```python
from build123d import *

# Parameters (mm, degrees)
SKETCH_1_W             = 94
SKETCH_1_H             = 94
EXTRUDE_1_DEPTH        = 30
FILLET_1_R             = 10
SHELL_1_T              = -2
SKETCH_2_W             = 24.1
SKETCH_2_H             = 30
EXTRUDE_3392_DEPTH     = 11
CUT_EXTRUDE_3513_REACH = 111.293
SKETCH_3_W             = 18.42
SKETCH_3_H             = 11.6
SKETCH_4_W             = 24.1
SKETCH_4_H             = 24.1
CUT_EXTRUDE_3826_DEPTH = 1.4
EXTRUDE_4548_DEPTH     = 14.2
SKETCH_9_W             = 69.4
SKETCH_9_H             = 9.2
SKETCH_10_W            = 5
SKETCH_10_H            = 5
EXTRUDE_5202_DEPTH     = 24.19
CUT_EXTRUDE_5310_DEPTH = 4
USBC_REACH             = 111.293
USBC_2_DEPTH           = 26
SKETCH_22_W            = 24.1
SKETCH_22_H            = 10.2
EXTRUDE_7617_DEPTH     = 24.95
CUT_EXTRUDE_6_REACH    = 70.81
SKETCH_23_R            = 2.2
SKETCH_23_R_2          = 3.7
SKETCH_13_W            = 10.3
SKETCH_13_H            = 10.3
EXTRUDE_4_DEPTH        = 28
CUT_EXTRUDE_7_DEPTH    = 4


with BuildPart() as part:
    # 草图1 → 凸台-拉伸1 (new body)
    with BuildSketch(Plane(origin=(0, 0, 0), x_dir=(1, 0, 0), z_dir=(0, 1, 0))):
        Rectangle(SKETCH_1_W, SKETCH_1_H)
    extrude(amount=EXTRUDE_1_DEPTH)

    # 圆角1
    fillet_1_edges = [part.edges().sort_by_distance(p)[0] for p in [
        (-47, 15, -47),
        (47, 15, -47),
        (47, 15, 47),
        (-47, 15, 47),
    ]]
    fillet(fillet_1_edges, radius=FILLET_1_R)

    # 抽壳1
    shell_1_openings = [part.faces().sort_by_distance(p)[0] for p in [
        (0, 0, 0),
    ]]
    offset(amount=SHELL_1_T, openings=shell_1_openings, kind=Kind.INTERSECTION)

    # 草图2 → Extrude 3392 (add)
    with BuildSketch(Plane.XY.offset(47)):
        with Locations((0, 15)):
            Rectangle(SKETCH_2_W, SKETCH_2_H)
    extrude(amount=-EXTRUDE_3392_DEPTH)

    # 草图3 → Cut-Extrude 3513 (cut, up to next)
    with BuildSketch(Plane.XY.offset(47), mode=Mode.PRIVATE) as cut_extrude_3513_sk1:
        with Locations((0, 12)):
            Rectangle(SKETCH_3_W, SKETCH_3_H)
    cut_extrude_3513_tool1 = extrude(cut_extrude_3513_sk1.sketch, amount=-CUT_EXTRUDE_3513_REACH, mode=Mode.PRIVATE) & part.part
    add(cut_extrude_3513_tool1.solids().sort_by_distance((0, 12, 47))[0], mode=Mode.SUBTRACT)

    # 草图4 → Cut-Extrude 3826 (cut)
    with BuildSketch(Plane.XZ.offset(-28)):
        with Locations((0, -1)):
            Rectangle(SKETCH_4_W, SKETCH_4_H)
    extrude(amount=-CUT_EXTRUDE_3826_DEPTH, mode=Mode.SUBTRACT)

    # 草图6 → Extrude 4548 (add)
    with BuildSketch(Plane.XZ.offset(-28)):
        with BuildLine():
            Line((-45, -37), (-45, -21.630094022))
            Line((-45, -21.630094022), (45, -21.630094022))
            Line((45, -21.630094022), (45, -37))
            ThreePointArc((45, -37), (42.656854249, -42.656854249), (37, -45))
            Line((37, -45), (-37, -45))
            ThreePointArc((-37, -45), (-42.656854249, -42.656854249), (-45, -37))
        make_face()
    extrude(amount=EXTRUDE_4548_DEPTH)

    # 草图9 → Cut-Revolve 4776 (revolve, cut)
    with BuildSketch(Plane.XZ.offset(-13.8)):
        with Locations((0, -31.2)):
            Rectangle(SKETCH_9_W, SKETCH_9_H)
    revolve(axis=Axis((-34.7, 13.8, -35.8), (1, 0, 0)), mode=Mode.SUBTRACT)

    # 草图10 → Extrude 5202 (add)
    with BuildSketch(Plane.XZ.offset(-28)):
        with Locations((-24, 23)):
            Rectangle(SKETCH_10_W, SKETCH_10_H)
        with Locations((24, -9)):
            Rectangle(SKETCH_10_W, SKETCH_10_H)
    extrude(amount=EXTRUDE_5202_DEPTH)

    # 草图11 → Cut-Extrude 5310 (cut)
    with BuildSketch(Plane.XZ.offset(-3.81)):
        Polygon((-23.076239569, 21.4), (-22.152479139, 23), (-23.076239569, 24.6), (-24.923760431, 24.6), (-25.847520861, 23), (-24.923760431, 21.4), align=None)
        Polygon((24.923760431, -10.6), (25.847520861, -9), (24.923760431, -7.4), (23.076239569, -7.4), (22.152479139, -9), (23.076239569, -10.6), align=None)
    extrude(amount=-CUT_EXTRUDE_5310_DEPTH, mode=Mode.SUBTRACT)

    # 草图15 → USBC (cut, up to next)
    with BuildSketch(Plane.XY.offset(47), mode=Mode.PRIVATE) as usbc_sk1:
        with BuildLine():
            Line((21.125, 13.6), (27.925, 13.6))
            ThreePointArc((27.925, 13.6), (29.525, 12), (27.925, 10.4))
            Line((27.925, 10.4), (21.125, 10.4))
            ThreePointArc((21.125, 10.4), (19.525, 12), (21.125, 13.6))
        make_face()
    usbc_tool1 = extrude(usbc_sk1.sketch, amount=-USBC_REACH, mode=Mode.PRIVATE) & part.part
    add(usbc_tool1.solids().sort_by_distance((24.525, 12, 47))[0], mode=Mode.SUBTRACT)

    # 草图16 → USBC 2 (add)
    with BuildSketch(Plane(origin=(0, 0, 45), x_dir=(-1, 0, 0), z_dir=(0, 0, -1))):
        Polygon((-15.225, 13), (-16.025, 13), (-16.025, 14.6), (-18.858333333, 14.6), (-18.858333333, 28), (-15.225, 28), align=None)
        Polygon((-30.191666667, 28), (-33.825, 28), (-33.825, 13), (-33.025, 13), (-33.025, 14.6), (-30.191666667, 14.6), align=None)
    extrude(amount=USBC_2_DEPTH)

    # 草图22 → Extrude 7617 (add)
    with BuildSketch(Plane(origin=(0, 0, 36), x_dir=(-1, 0, 0), z_dir=(0, 0, -1))):
        with Locations((0, 22.9)):
            Rectangle(SKETCH_22_W, SKETCH_22_H)
    extrude(amount=EXTRUDE_7617_DEPTH)

    # 草图23 → 切除-拉伸6 (cut, up to next)
    with BuildSketch(Plane(origin=(0, 17.8, 0), x_dir=(-1, 0, 0), z_dir=(0, -1, 0)), mode=Mode.PRIVATE) as cut_extrude_6_sk1:
        with Locations(Location((0, -32, 0), (0, 0, 180))):
            Circle(SKETCH_23_R)
    cut_extrude_6_tool1 = extrude(cut_extrude_6_sk1.sketch, amount=-CUT_EXTRUDE_6_REACH, mode=Mode.PRIVATE) & part.part
    # 草图23 → 切除-拉伸6 (cut, up to next)
    with BuildSketch(Plane(origin=(0, 17.8, 0), x_dir=(-1, 0, 0), z_dir=(0, -1, 0)), mode=Mode.PRIVATE) as cut_extrude_6_sk2:
        with Locations(Location((0, -22, 0), (0, 0, 180))):
            Circle(SKETCH_23_R_2)
    cut_extrude_6_tool2 = extrude(cut_extrude_6_sk2.sketch, amount=-CUT_EXTRUDE_6_REACH, mode=Mode.PRIVATE) & part.part
    add(cut_extrude_6_tool1.solids().sort_by_distance((0, 17.8, 32))[0], mode=Mode.SUBTRACT)
    add(cut_extrude_6_tool2.solids().sort_by_distance((0, 17.8, 22))[0], mode=Mode.SUBTRACT)

    # 草图13 → 凸台-拉伸4 (add)
    with BuildSketch(Plane.XZ.offset(-28)):
        with BuildLine():
            Line((-45, -37), (-45, -16.768109074))
            Line((-45, -16.768109074), (-34.7, -16.768109074))
            Line((-34.7, -16.768109074), (-34.7, -45))
            Line((-34.7, -45), (-37, -45))
            ThreePointArc((-37, -45), (-42.656854249, -42.656854249), (-45, -37))
        make_face()
        with BuildLine():
            Line((34.7, -16.768109074), (34.7, -45))
            Line((34.7, -45), (37, -45))
            ThreePointArc((37, -45), (42.656854249, -42.656854249), (45, -37))
            Line((45, -37), (45, -16.768109074))
            Line((45, -16.768109074), (34.7, -16.768109074))
        make_face()
        with Locations((-39.85, 31.85)):
            Rectangle(SKETCH_13_W, SKETCH_13_H)
        with Locations((39.85, 31.85)):
            Rectangle(SKETCH_13_W, SKETCH_13_H)
    extrude(amount=EXTRUDE_4_DEPTH)

    # 草图26 → 切除-拉伸7 (cut)
    with BuildSketch(Plane.XZ):
        Polygon((-40.85, 30.117949192), (-38.85, 30.117949192), (-37.85, 31.85), (-38.85, 33.582050808), (-40.85, 33.582050808), (-41.85, 31.85), align=None)
        Polygon((40.85, 33.582050808), (41.85, 31.85), (40.85, 30.117949192), (38.85, 30.117949192), (37.85, 31.85), (38.85, 33.582050808), align=None)
        Polygon((40.85, -23.267949192), (41.85, -25), (40.85, -26.732050808), (38.85, -26.732050808), (37.85, -25), (38.85, -23.267949192), align=None)
        Polygon((-40.85, -23.267949192), (-41.85, -25), (-40.85, -26.732050808), (-38.85, -26.732050808), (-37.85, -25), (-38.85, -23.267949192), align=None)
    extrude(amount=-CUT_EXTRUDE_7_DEPTH, mode=Mode.SUBTRACT)


solid = part.part
```
For this review, take the finished solid that the model builds, in its own axes (mm). A direction names the side the tool comes from. Round coordinates to 2 decimals unless told otherwise and drop trailing zeros. Write each loop counter-clockwise with the first axis right and the second up, starting at its lowest first coordinate (ties: lowest second). Pieces come first, ordered by that corner, then holes. Notation, with made-up numbers: (30, 15.5) -> (82, 15.5) arc R21 ccw to (82, 38.5) -> close; hole circle Ø6 at (59, 44). An arc over 180 degrees is marked (long way). One line per question, with ' | ' between items. Start each with the question number.
(1) Mouldability with a two-part tool opening along X and no side actions: class faces 1 (the face through (26.5, 16, -9)), 2 (the face through (44.15, 15.21, -43.99)), 3 (the face through (-1, 19, 47)), 4 (the face through (0, 29.4, -1)) as released by +X, released by -X, zero draft, split by the parting line, or undercut.
(2) Add section A-A, the plane x = 0. Write out the cut boundary in (y, z), plus the area to 3 significant figures.
(3) Add section D-D, the plane z = -1. Write out the cut boundary in (x, y), plus the area to 3 significant figures.
(4) Add section C-C, the plane y = 20.75. Give the number of separate pieces and of enclosed holes in the cut face, plus the area to 3 significant figures.
(5) Tool access review of faces 5 (the face through (-24, 3.81, 25)), 6 (the face through (9.21, 12, 42)), 7 (the face through (1.71, 23.81, 18.72)): name each direction out of +Z, -Z, +X, -X, +Y, -Y from which nothing blocks a thin tool from reaching the whole face with its end or side.
(6) Insertion check: P1, Ø20, axis at x = 1, z = 20, coming from the -Y side; P2, Ø5, axis at x = -38, y = 19.5, coming from the +Z side; P3, Ø2, axis at x = 40, y = 2, coming from the -Z side; P4, Ø5.5, axis at y = 9.5, z = 41.5, coming from the -X side. Each pin has a flat end and moves straight along its axis. Give the tip position at first contact, or say it passes through.
(7) For line 1 along Z through (x, y) = (-36, 22.75); line 2 along Z through (x, y) = (24.5, 23.5); line 3 along Z through (x, y) = (0, 26.5), list the stretches that pass through material, from the lowest coordinate up. Write a range as from..to.
(8) Add section B-B, the plane z = -14.5. Write out the cut boundary in (x, y).
Answer list:
1) face 1: undercut | face 2: released by +X | face 3: zero draft | face 4: undercut
2) outline: (0, -47) -> (30, -47) -> (30, 18.3) -> (17.8, 18.3) -> (17.8, 11.05) -> (29.4, 11.05) -> (29.4, -13.05) -> (28, -13.05) -> (28, -21.63) -> (13.8, -21.63) -> (13.8, -26.6) arc R9.2 cw to (13.8, -45) -> (0, -45) -> close; (0, 36) -> (6.2, 36) -> (6.2, 47) -> (0, 47) -> close; (17.8, 25.7) -> (30, 25.7) -> (30, 29.8) -> (17.8, 29.8) -> close; (17.8, 34.2) -> (30, 34.2) -> (30, 47) -> (17.8, 47) -> close | area: 700 mm²
3) outline: (-47, 0) -> (-45, 0) -> (-45, 28) -> (-12.05, 28) -> (-12.05, 29.4) -> (12.05, 29.4) -> (12.05, 28) -> (45, 28) -> (45, 0) -> (47, 0) -> (47, 30) -> (-47, 30) -> close | area: 266 mm²
4) separate pieces: 3 | enclosed holes: 4 | area: 3,260 mm²
5) face 5: -Y | face 6: +Z | face 7: +Y, -Y
6) P1: y = 17.8 | P2: z = 47 | P3: z = -46.8 | P4: x = -46.85
7) line 1: -47..-16.77, 26.7..37, 45..47 | line 2: -47..-21.63, -11.5..-6.5, 45..47 | line 3: -47..-21.63, 11.05..18.3, 25.7..29.8, 34.2..47
8) outline: (-47, 0) -> (-45, 0) -> (-45, 28) -> (45, 28) -> (45, 0) -> (47, 0) -> (47, 30) -> (-47, 30) -> close
